Could you check a few things on this model? Use its own coordinates, in mm. A direction names the side the tool comes from. Give positions to 0.01 mm unless a question says otherwise; leave off trailing zeros. Write each loop counter-clockwise with the first axis right and the second up, starting at its lowest first coordinate (ties: lowest second). Pieces come first, ordered by that corner, then holes. Notation, with made-up numbers: M 59.5,89 L 112.5,89 A11 cw 112.5,103 Z; hole C 82,-18.5 d10. An arc over 180 degrees is marked long. Answer as CSV lines item,"result". Start each with the question number.
from build123d import *

# Parameters (mm, degrees)
BOSS_EXTRUDE2_DEPTH = 3.18
SKETCH8_R           = 3.25
BOSS_EXTRUDE3_DEPTH = 3.18
FILLET4_R           = 2
FILLET5_R           = 1
SKETCH9_R           = 2.39
CUT_EXTRUDE1_DEPTH  = 3.18
FILLET6_R           = 2
FILLET7_R           = 2
FILLET8_R           = 2
BOSS_EXTRUDE6_DEPTH = 10
SKETCH12_R          = 7.894491475
CUT_EXTRUDE2_DEPTH  = 20


with BuildPart() as part:
    # Sketch1 → Boss-Extrude2 (new body)
    with BuildSketch(Plane(origin=(0, 0, 0), x_dir=(1, 0, 0), z_dir=(0, 1, 0))):
        Polygon((0, 0), (0, 50), (13, 50), (13, 41.521912351), (63, 41.521912351), (63, 50), (76, 50), (76, 0), (63, 0), (63, 14.685258964), (51.88, 14.685258964), (51.88, 6.566903426), (24.12, 6.566903426), (24.12, 14.685258964), (13, 14.685258964), (13, 0), align=None)
    extrude(amount=-BOSS_EXTRUDE2_DEPTH)

    # Sketch8 → Boss-Extrude3 (add)
    with BuildSketch(Plane.XY.offset(-6.566903426)):
        with BuildLine():
            Line((24.12, -45.5), (24.12, -20.153398116))
            Line((24.12, -20.153398116), (24.12, 0))
            Line((24.12, 0), (51.879574545, 0))
            Line((51.879574545, 0), (51.879574545, -17.65))
            Line((51.879574545, -17.65), (60.204359999, -21.94))
            Line((60.204359999, -21.94), (60.204359999, -43.21))
            Line((60.204359999, -43.21), (51.879574545, -47.5))
            Line((51.879574545, -47.5), (26.12, -47.5))
            ThreePointArc((26.12, -47.5), (24.705786438, -46.914213562), (24.12, -45.5))
        make_face()
        with Locations((38.348750497, -25.08)):
            Circle(SKETCH8_R, mode=Mode.SUBTRACT)
        with Locations((38.348750497, -40.08)):
            Circle(SKETCH8_R, mode=Mode.SUBTRACT)
        with BuildLine():
            Line((57.524359999, -23.223501404), (57.524359999, -28.546918648))
            ThreePointArc((57.524359999, -28.546918648), (55.134359999, -30.936918648), (52.744359999, -28.546918648))
            Line((52.744359999, -28.546918648), (52.744359999, -23.223501404))
            ThreePointArc((52.744359999, -23.223501404), (55.134359999, -20.833501404), (57.524359999, -23.223501404))
        make_face(mode=Mode.SUBTRACT)
        with BuildLine():
            Line((57.524359999, -36.223501404), (57.524359999, -41.546918648))
            ThreePointArc((57.524359999, -41.546918648), (55.134359999, -43.936918648), (52.744359999, -41.546918648))
            Line((52.744359999, -41.546918648), (52.744359999, -36.223501404))
            ThreePointArc((52.744359999, -36.223501404), (55.134359999, -33.833501404), (57.524359999, -36.223501404))
        make_face(mode=Mode.SUBTRACT)
    extrude(amount=BOSS_EXTRUDE3_DEPTH)

    # Fillet4
    fillet4_edges = [part.edges().sort_by_distance(p)[0] for p in [
        (37.999787272, 0, -3.386903426),
    ]]
    fillet(fillet4_edges, radius=FILLET4_R)

    # Fillet5
    fillet5_edges = [part.edges().sort_by_distance(p)[0] for p in [
        (37.999787272, -3.18, -6.566903426),
    ]]
    fillet(fillet5_edges, radius=FILLET5_R)

    # Sketch9 → Cut-Extrude1 (cut)
    with BuildSketch(Plane(origin=(0, 0, 0), x_dir=(1, 0, 0), z_dir=(0, 1, 0))):
        with Locations((6.5, 5)):
            Circle(SKETCH9_R)
        with Locations((6.5, 20)):
            Circle(SKETCH9_R)
        with Locations((69.5, 20)):
            Circle(SKETCH9_R)
        with Locations((69.5, 5)):
            Circle(SKETCH9_R)
    extrude(amount=-CUT_EXTRUDE1_DEPTH, mode=Mode.SUBTRACT)

    # Fillet6
    fillet6_edges = [part.edges().sort_by_distance(p)[0] for p in [
        (0, -1.59, 0),
    ]]
    fillet(fillet6_edges, radius=FILLET6_R)

    # Fillet7
    fillet7_edges = [part.edges().sort_by_distance(p)[0] for p in [
        (13, -1.59, 0),
    ]]
    fillet(fillet7_edges, radius=FILLET7_R)

    # Fillet8
    fillet8_edges = [part.edges().sort_by_distance(p)[0] for p in [
        (0, -1.59, -50),
        (13, -1.59, -50),
        (13, -1.59, -41.521912351),
        (63, -1.59, -41.521912351),
        (63, -1.59, -50),
        (76, -1.59, -50),
        (76, -1.59, 0),
        (63, -1.59, 0),
        (63, -1.59, -14.685258964),
        (51.88, -1.59, -14.685258964),
        (24.12, -1.59, -14.685258964),
        (13, -1.59, -14.685258964),
    ]]
    fillet(fillet8_edges, radius=FILLET8_R)

    # Sketch11 → Boss-Extrude6 (add, symmetric)
    with BuildSketch(Plane(origin=(38, 0, 0), x_dir=(0, 0, -1), z_dir=(1, 0, 0))):
        Polygon((25, -3.18), (6.54535076, -3.18), (6.54535076, -21.63464924), align=None)
    extrude(amount=BOSS_EXTRUDE6_DEPTH, both=True)

    # Sketch12 → Cut-Extrude2 (cut)
    with BuildSketch(Plane(origin=(0, 0, -6.566903426), x_dir=(-1, 0, 0), z_dir=(0, 0, -1))):
        with Locations((-38.348750497, -25.08)):
            Circle(SKETCH12_R)
    extrude(amount=CUT_EXTRUDE2_DEPTH, mode=Mode.SUBTRACT)


solid = part.part
1. Imagine slicing it at D-D, the plane z = -20. Please give me the cut outline in (x, y).
2. On a 3-axis mill with a long thin cutter (end or side, diameter ignored), from which of +Z, -Z, +X, -X, +Y, -Y can I reach the whole of each face in a straight line? I mean faces 1 (the cylindrical face through (62.399, -1.612, -42.092)), 2 (the cylindrical face through (63.6, -1.61, -0.57)), 3 (the flat face through (48, -10, -14)). Say none if no direction works.
3. Please list where these lines run through material, in increasing order: line 1 (Z direction, x = 6.5, y = -1.6); line 2 (X direction, y = -2.4, z = -5); line 3 (Y direction, x = 20, z = -36).
4. Imagine slicing it at B-B, the plane z = -46. Please give me the cut outline in (x, y), plus the area to 3 significant figures.
5. Thinking about a two-plate mould opening in X: for faces 4 (the cylindrical face through (12.4, -1.61, -49.43)), 5 (the flat face through (38.5, -3.18, -25.4)), 6 (the cylindrical face through (24.72, -46.93, -5)), which applies, pulls with the +X half, pulls with the -X half, needs draft (parallel to the pull), parting line crosses it, or undercut?
6. Will these pins go through, and if not, where does the flat tip stop? P1, Ø6, axis at x = 46.5, z = -39, coming from the +Y side; P2, Ø5, axis at x = 38.35, y = -40.08, coming from the -Z side; P3, Ø1, axis at y = -26.5, z = -5.5, coming from the -X side; P4, Ø6, axis at x = 35.5, z = -38.5, coming from the -Y side.
7. Imagine slicing it at A-A, the plane y = -25.08. Please give me the cut outline in (x, z).
8. Imagine slicing it at C-C, the plane x = 69.5. Please give me the cut outline in (y, z).
Solutions:
1,outline,"M 0,-3.18 L 4.11,-3.18 L 4.11,0 L 0,0 Z; M 8.89,-3.18 L 28,-3.18 L 28,-8.18 L 48,-8.18 L 48,-3.18 L 67.11,-3.18 L 67.11,0 L 8.89,0 Z; M 71.89,-3.18 L 76,-3.18 L 76,0 L 71.89,0 Z"
2,face 1,"-Z, +Y, -Y"
2,face 2,"+Z, +Y, -Y"
2,face 3,"-Z, +X, -Y"
3,line 1,"-50 to -22.39, -17.61 to -7.39, -2.61 to 0"
3,line 2,"0 to 4.11, 8.89 to 13, 24.12 to 51.88, 63 to 67.11, 71.89 to 76"
3,line 3,"-3.18 to 0"
4,outline,"M 0,-3.18 L 13,-3.18 L 13,0 L 0,0 Z; M 63,-3.18 L 76,-3.18 L 76,0 L 63,0 Z"
4,area,"82.7 mm²"
5,face 4,"undercut"
5,face 5,"needs draft"
5,face 6,"pulls with the -X half"
6,P1,"y = 0"
6,P2,"through"
6,P3,"x = 24.12"
6,P4,"y = -3.18"
7,outline,"M 24.12,-6.57 L 35.1,-6.57 L 35.1,-3.39 L 24.12,-3.39 Z; M 41.6,-6.57 L 52.74,-6.57 L 52.74,-3.39 L 41.6,-3.39 Z; M 57.52,-6.57 L 60.2,-6.57 L 60.2,-3.39 L 57.52,-3.39 Z"
8,outline,"M -3.18,-50 L 0,-50 L 0,-22.39 L -3.18,-22.39 Z; M -3.18,-17.61 L 0,-17.61 L 0,-7.39 L -3.18,-7.39 Z; M -3.18,-2.61 L 0,-2.61 L 0,0 L -3.18,0 Z"
